Check sheet for the modelled part. Datum: model origin and axes. Units: mm. A direction names the side the tool comes from. Round coordinates to 2 decimals unless told otherwise and drop trailing zeros. Write each loop counter-clockwise with the first axis right and the second up, starting at its lowest first coordinate (ties: lowest second). Pieces come first, ordered by that corner, then holes. Notation, with made-up numbers: M 2,49.5 L 49,49.5 A14 ccw 49,58.5 Z; hole C 36,28 d8. An arc over 180 degrees is marked long. One line per item, written item: value.
from build123d import *

# Parameters (mm, degrees)
BOSS_EXTRUDE1_DEPTH = 19


with BuildPart() as part:
    # Sketch1 → Boss-Extrude1 (new body)
    with BuildSketch(Plane.XY):
        Polygon((-21.15, 14.15), (-14.15, 21.15), (14.15, 21.15), (21.15, 14.15), (21.15, -14.15), (14.15, -21.15), (-14.15, -21.15), (-21.15, -14.15), align=None)
        Polygon((-12.078932188, 16.15), (12.078932188, 16.15), (16.15, 12.078932188), (16.15, -12.078932188), (12.078932188, -16.15), (-12.078932188, -16.15), (-16.15, -12.078932188), (-16.15, 12.078932188), align=None, mode=Mode.SUBTRACT)
    extrude(amount=BOSS_EXTRUDE1_DEPTH)


solid = part.part
Q1. Access from +Z, -Z, +X, -X, +Y, -Y to the whole of each face (thin tool, end or side, straight path). Record for faces 1 (the flat face through (-17.7, 17.6, 9.4)), 2 (the flat face through (0, 16.15, 9)).
Completed:
face 1: +Z, -Z, -X, +Y
face 2: +Z, -Z
Q2. Sectioned sample at D-D on y = 17.5. Enter the section's corners in (x, z), and give its area (3 significant figures).
Completed:
outline: M -17.8,0 L 17.8,0 L 17.8,19 L -17.8,19 Z
area: 676 mm^2
Q3. Sectioned sample at A-A on x = -10. Enter the section's corners in (y, z), and give its area (3 significant figures).
Completed:
outline: M -21.15,0 L -16.15,0 L -16.15,19 L -21.15,19 Z; M 16.15,0 L 21.15,0 L 21.15,19 L 16.15,19 Z
area: 190 mm^2
Q4. Depth check by flat-ended pin: P1, Ø4, axis at y = 17, z = 10.5, coming from the -X side. Enter the tip coordinate at first touch or a pass-through.
Completed:
P1: x = -20.3
Q5. Draft check along Y on faces 3 (the flat face through (-16.15, 0, 9)), 4 (the flat face through (17.7, -17.6, 9.4)), 5 (the flat face through (17, 2, 19)). Enter one of: pulls with the +Y half, pulls with the -Y half, needs draft (parallel to the pull), parting line crosses it, or undercut.
Completed:
face 3: undercut
face 4: pulls with the -Y half
face 5: needs draft
Q6. Sectioned sample at C-C on z = 11.25. Enter the section's corners in (x, y).
Completed:
outline: M -21.15,-14.15 L -14.15,-21.15 L 14.15,-21.15 L 21.15,-14.15 L 21.15,14.15 L 14.15,21.15 L -14.15,21.15 L -21.15,14.15 Z; hole M -16.15,-12.08 L -12.08,-16.15 L 12.08,-16.15 L 16.15,-12.08 L 16.15,12.08 L 12.08,16.15 L -12.08,16.15 L -16.15,12.08 Z
Q7. Scan lines: line 1 (X direction, y = 3, z = 14); line 2 (Y direction, x = -13, z = 9.5). Record each from-to range of solid material in increasing order. Write a range as [from, to].
Completed:
line 1: [-21.15, -16.15], [16.15, 21.15]
line 2: [-21.15, -15.23], [15.23, 21.15]
